Can you work these out from the drawing? Everything is in mm from the part's minimum corner. A direction names the side the tool comes from. Coordinates: 2 decimals unless noted, no trailing zeros. Order: outer loops, then holes, each group sorted by start corner. A loop starts at its lowest first (then second) coordinate and runs counter-clockwise, first axis right, second up. Notation, with made-up numbers: (-39, -2.5) -> (-17, -2.5) arc R11 ccw to (-17, 6.5) -> close; hole circle Ø5 at (7, -22.5). An arc over 180 degrees is marked (long way). Put each result on its own line as item: value. Start each with the question number.
Q1. Please list where these lines run through material, in increasing order: line 1 along X through (y, z) = (1, 2) (1 decimal); line 2 along Z through (x, y) = (1.5, 7) (1 decimal); line 3 along Y through (x, z) = (2.25, 3.5) (1 decimal).
Q2. We'd pull the mould along X, two halves only. Please class the marked faces 1, 2 and 3: +X half, -X half, draft (parallel to the pull), parting line (faces both ways), or undercut.
Q3. If we section it at C-C (x = 1): Please give me the cut outline in (y, z) (1 decimal).
Q4. Will these pins go through, and if not, where does the flat tip stop? pin 1 (4.5 mm diameter, centred on x = 6.5, y = 8, fed in from -Z); pin 2 (1 mm diameter, centred on x = 2.5, z = 4, fed in from -Y); pin 3 (2 mm diameter, centred on x = 4.5, z = 4, fed in from +Y).
Q5. For the marked faces 4, 5 and 6, which set-ups out of +Z, -Z, +X, -X, +Y, -Y let a thin tool reach every point of the face, with its end or its side?
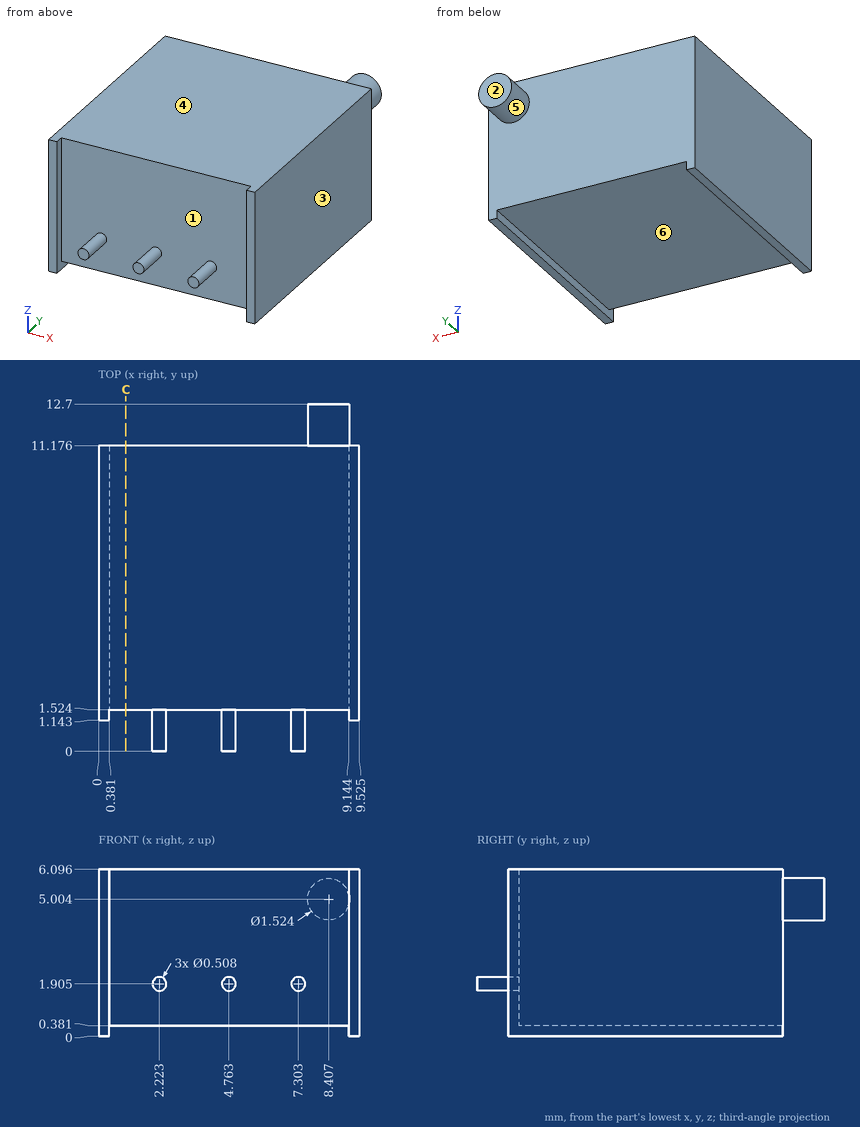
The answers:
1. line 1: 2 to 2.5, 4.5 to 5, 7.1 to 7.5
1. line 2: 0.4 to 6.1
1. line 3: 1.5 to 11.2
2. face 1: undercut
2. face 2: draft
2. face 3: +X half
3. outline: (1.5, 0.4) -> (11.2, 0.4) -> (11.2, 6.1) -> (1.5, 6.1) -> close
4. pin 1: z = 0.38
4. pin 2: y = 1.52
4. pin 3: y = 11.18
5. face 4: +Z, +X, -X, +Y, -Y
5. face 5: +Y
5. face 6: -Z, +Y, -Y
